```python
from build123d import *

# Parameters (mm, degrees)
F0_W     = 600
F0_H     = 100
F1_DEPTH = 20
F2_W     = 20
F2_H     = 20
F3_DEPTH = 20
F4_W     = 600
F4_H     = 10
F5_DEPTH = 10


with BuildPart() as f1:
    # F0 (on Front) → F1 (new body)
    with BuildSketch(Plane.XZ):
        Rectangle(F0_W, F0_H)
    extrude(amount=F1_DEPTH)

    # F2 (on face) → F3 (cut, through all)
    with BuildSketch(Plane(origin=(0, 0, 0), x_dir=(-1, 0, 0), z_dir=(0, 1, 0))):
        with Locations((-290, -40)):
            Rectangle(F2_W, F2_H)
        with Locations((-290, 0)):
            Rectangle(F2_W, F2_H)
        with Locations((290, 0)):
            Rectangle(F2_W, F2_H)
        with Locations((290, -40)):
            Rectangle(F2_W, F2_H)
        with Locations((290, 40)):
            Rectangle(F2_W, F2_H)
        with Locations((-290, 40)):
            Rectangle(F2_W, F2_H)
    extrude(amount=-F3_DEPTH, mode=Mode.SUBTRACT)

    # F4 (on face) → F5 (cut)
    with BuildSketch(Plane.XZ.offset(20)):
        with Locations((0, 35)):
            Rectangle(F4_W, F4_H)
    extrude(amount=-F5_DEPTH, mode=Mode.SUBTRACT)


solid = f1.part
```
Could you check a few things on this model? Use its own coordinates, in mm. A direction names the side the tool comes from. Give positions to 0.01 mm unless a question says otherwise; leave off trailing zeros. Loops run counter-clockwise (first coordinate to the right, second up) from the corner with the lowest first, then second, coordinate; pieces in that order, holes last. Notation, with made-up numbers: (43.25, -10.75) - (67.25, -10.75) arc R14 cw to (67.25, 2.25) - close; hole circle Ø2 at (68, 21.25). An arc over 180 degrees is marked (long way). Use one line per item in the form item = value.
1. I'm going to push flat-ended pins straight in: pin 1 Ø10 at (x, y) = (285.5, -6) entering from -Z; pin 2 Ø3 at (x, z) = (50.5, 36) entering from -Y; pin 3 Ø6 at (y, z) = (-10, 3.5) entering from -X. Where does each tip first touch, or does it pass through?
Response values:
pin_1 = -30
pin_2 = -10
pin_3 = -280
2. I want a section at C-C (z = -35.5). Please give me the cut outline in (x, y).
Response values:
outline = (-280, -20) - (280, -20) - (280, 0) - (-280, 0) - close
3. I need wall thicknesses on probe 1 along Z at (x, y) = (-115, -12.5); probe 2 along Y at (x, z) = (-135, 33); probe 3 along X at (y, z) = (-3, -38). Which ranges of each line are inside material? Lowest first, please.
Response values:
probe_1 = -50 to 30, 40 to 50
probe_2 = -10 to 0
probe_3 = -280 to 280
4. On a 3-axis mill with a long thin cutter (end or side, diameter ignored), from which of +Z, -Z, +X, -X, +Y, -Y can I reach the whole of each face in a straight line? I mean faces 1 (the face through (290, -10, -30)), 2 (the face through (-4, -10, 35)), 3 (the face through (290, -10, 10)), 4 (the face through (-280, -10, 0)). Say none if no direction works.
Response values:
face_1 = -Z, +X, +Y, -Y
face_2 = +X, -X, -Y
face_3 = +X, +Y, -Y
face_4 = -X, +Y, -Y
5. I want a section at B-B (x = 252.5). Please give me the cut outline in (y, z).
Response values:
outline = (-20, -50) - (0, -50) - (0, 50) - (-20, 50) - (-20, 40) - (-10, 40) - (-10, 30) - (-20, 30) - close
6. I want a section at A-A (y = -13.5). Please give me the cut outline in (x, z).
Response values:
outline = (-300, -30) - (-280, -30) - (-280, -50) - (280, -50) - (280, -30) - (300, -30) - (300, -10) - (280, -10) - (280, 10) - (300, 10) - (300, 30) - (-300, 30) - (-300, 10) - (-280, 10) - (-280, -10) - (-300, -10) - close; (-280, 40) - (280, 40) - (280, 50) - (-280, 50) - close
7. Thinking about a two-plate mould opening in Z: for faces 5 (the face through (290, -10, -10)), 6 (the face through (-4, -10, -50)), 7 (the face through (-4, 0, 1)), which applies, released by +Z, released by -Z, zero draft, split by the parting line, or undercut?
Response values:
face_5 = undercut
face_6 = released by -Z
face_7 = zero draft
